```python
from build123d import *

# Parameters (mm, degrees)
SKETCH_1_R               = 8.6
EXTRUDE_1_DEPTH          = 17.7
SKETCH_2_R               = 3.05
SKETCH_2_R_2             = 2.55
EXTRUDE_2_DEPTH          = 1.5
SHELL_4_OUTLINE_R        = 7.6
SHELL_4_DEPTH            = 16.7
SHELL_START              = 16.7
SHELL_4_2_OUTLINE_R      = 2.05
SHELL_4_2_DEPTH          = 1
SKETCH_5_R               = 0.8
SKETCH_5_R_2             = 0.5
SKETCH_5_W               = 1.5
SKETCH_5_H               = 1
CUT_EXTRUDE_5_DEPTH      = 1.5
CUT_EXTRUDE_6_DEPTH      = 0.5
PATTERN_CIRCULAR_1_COUNT = 4
FILLET_1_R               = 0.5


# Read off the part's stored shape, not the designer's step: 薄殼4
with BuildPart() as part:
    # 草圖1 → 伸長1 (new body)
    with BuildSketch(Plane(origin=(0, 0, 0), x_dir=(1, 0, 0), z_dir=(0, 1, 0))):
        with Locations(Location((0, 0, 0), (0, 0, 270))):
            Circle(SKETCH_1_R)
    extrude(amount=EXTRUDE_1_DEPTH)

    # 草圖2 → 伸長2 (add)
    with BuildSketch(Plane(origin=(0, 17.7, 0), x_dir=(1, 0, 0), z_dir=(0, 1, 0))):
        with Locations(Location((0, 0, 0), (0, 0, 270))):
            Circle(SKETCH_2_R)
        with Locations(Location((0, 0, 0), (0, 0, 270))):
            Circle(SKETCH_2_R_2, mode=Mode.SUBTRACT)
    extrude(amount=EXTRUDE_2_DEPTH)

    # 薄殼4 outline → 薄殼4 (cut)
    with BuildSketch(Plane(origin=(0, 0, 0), x_dir=(1, 0, 0), z_dir=(0, 1, 0))):
        Circle(SHELL_4_OUTLINE_R)
    extrude(amount=SHELL_4_DEPTH, mode=Mode.SUBTRACT)

    # Shell 4 2 outline → Shell 4 2 (cut)
    with BuildSketch(Plane(origin=(0, 0, 0), x_dir=(1, 0, 0), z_dir=(0, 1, 0)).offset(SHELL_START)):
        Circle(SHELL_4_2_OUTLINE_R)
    extrude(amount=SHELL_4_2_DEPTH, mode=Mode.SUBTRACT)

    # 草圖5 → 伸長5 (cut)
    with BuildSketch(Plane(origin=(0, 17.7, 0), x_dir=(1, 0, 0), z_dir=(0, 1, 0))):
        with Locations(Location((-5.5, 3.175426481, 0), (0, 0, 270))):
            Circle(SKETCH_5_R)
        with Locations(Location((-5.75, 0, 0), (0, 0, 270))):
            Circle(SKETCH_5_R_2)
        with Locations(Location((5.75, 0, 0), (0, 0, 270))):
            Circle(SKETCH_5_R_2)
        with Locations((0, 7.75)):
            Rectangle(SKETCH_5_W, SKETCH_5_H)
        with Locations((0, -7.75)):
            Rectangle(SKETCH_5_W, SKETCH_5_H)
    extrude(amount=-CUT_EXTRUDE_5_DEPTH, mode=Mode.SUBTRACT)

    # 草圖7 → 伸長6 (cut)
    with BuildSketch(Plane.XZ):
        Polygon((-5.762920267, 4.348706704), (-6.965001795, 5.550788232), (-5.550788232, 6.965001795), (-4.348706704, 5.762920267), align=None)
    cut_extrude_6 = extrude(amount=-CUT_EXTRUDE_6_DEPTH, mode=Mode.SUBTRACT)

    # 環狀複製排列1: 伸長6 ×4 about axis
    pattern_circular_1_axis = Axis((0, 0, 0), (0, 1, 0))
    for i in range(1, PATTERN_CIRCULAR_1_COUNT):
        add(cut_extrude_6.rotate(pattern_circular_1_axis, i * 360 / PATTERN_CIRCULAR_1_COUNT), mode=Mode.SUBTRACT)

    # 圓角1
    # the kernel refuses this fillet: 0.5 mm, written as the material it takes off along each edge
    with BuildSketch(Plane(origin=(0, 17.7, 0), x_dir=(0, 0, 1), z_dir=(-1, 0, 0))) as fillet_1_piece_1:
        with BuildLine():
            CenterArc((8.6 - FILLET_1_R, -FILLET_1_R), FILLET_1_R, 0, 90)
            Line((8.6 - FILLET_1_R, 0), (8.6, 0))
            Line((8.6, 0), (8.6, -FILLET_1_R))
        make_face()
    revolve(axis=Axis((0, 17.7, 0), (0, 1, 0)), mode=Mode.SUBTRACT)


solid = part.part
```
Input: part model. Units: mm. Frame: model coordinates. A direction names the side the tool comes from. Coordinates: 2 decimals unless noted, no trailing zeros. Loops run counter-clockwise (first coordinate to the right, second up) from the corner with the lowest first, then second, coordinate; pieces in that order, holes last. Notation, with made-up numbers: M 59,-26 L 93,-26 A26 cw 93,-7 Z; hole C -38,-10 d8. An arc over 180 degrees is marked long. Use a Markdown table: item, result. Add a question column.
1) Section A-A, the plane z = 0. Give the number of separate pieces and of enclosed holes in the cut face, plus the area to 3 significant figures.
2) Section B-B, the plane x = 0. Return the cut outline in (y, z).
3) Pin query (flat end, axial travel): P1, Ø5.5, axis at x = 0, z = 0, coming from the -Y side; P2, Ø5, axis at x = -5.5, y = 10.5, coming from the +Z side; P3, Ø1.1, axis at y = 17, z = -7.5, coming from the +X side. Return the tip coordinate at first contact, or that it passes through.
4) Draft query along Z for faces 1 (the flat face through (-2, 19.2, 2)), 2 (the cylindrical face through (-1.856, 18.44, -2.42)), 3 (the flat face through (-0.75, 17, -8)). Return one class per face: +Z half, -Z half, draft (parallel to the pull), parting line (faces both ways), or undercut.
5) Section C-C, the plane y = 13.25. Return the cut outline in (x, z).
6) Set-up query: faces 4 (the flat face through (0, 17, 7.25)), 5 (the flat face through (-5.9, 0.5, 5.7)), 6 (the flat face through (0.75, 17, 8)). Return all of +Z, -Z, +X, -X, +Y, -Y with unobstructed straight access to the full face (end or side cutting, diameter ignored); none if empty.
7) Line query: L1, parallel to Z at x = 0, y = 17.4; L2, parallel to Z at x = 0, y = 17.5; L3, parallel to X at y = 17.45, z = 0. Output: solid intervals per line, ascending. Write a range as from..to.
Answer below:
| question | item | result |
|---|---|---|
| 1 | separate pieces | 4 |
| 1 | enclosed holes | 0 |
| 1 | area | 45.9 mm2 |
| 2 | outline | M 0,-8.6 L 17.2,-8.6 A0.5 ccw 17.68,-8.25 L 16.2,-8.25 L 16.2,-7.6 L 0,-7.6 Z; M 0,7.6 L 16.2,7.6 L 16.2,8.25 L 17.68,8.25 A0.5 ccw 17.2,8.6 L 0,8.6 Z; M 16.7,-7.25 L 17.7,-7.25 L 17.7,-3.05 L 19.2,-3.05 L 19.2,-2.55 L 17.7,-2.55 L 17.7,-2.05 L 16.7,-2.05 Z; M 16.7,2.05 L 17.7,2.05 L 17.7,2.55 L 19.2,2.55 L 19.2,3.05 L 17.7,3.05 L 17.7,7.25 L 16.7,7.25 Z |
| 3 | P1 | y = 16.7 |
| 3 | P2 | z = 8.06 |
| 3 | P3 | x = 5.07 |
| 4 | face 1 | draft |
| 4 | face 2 | parting line |
| 4 | face 3 | undercut |
| 5 | outline | C 0,0 d17.2; hole C 0,0 d15.2 |
| 6 | face 4 | +Y, -Y |
| 6 | face 5 | -Y |
| 6 | face 6 | +Y |
| 7 | L1 | -8.56..-8.25, -7.25..-2.05, 2.05..7.25, 8.25..8.56 |
| 7 | L2 | -8.5..-8.25, -7.25..-2.05, 2.05..7.25, 8.25..8.5 |
| 7 | L3 | -8.53..-6.25, -5.25..-2.05, 2.05..5.25, 6.25..8.53 |
